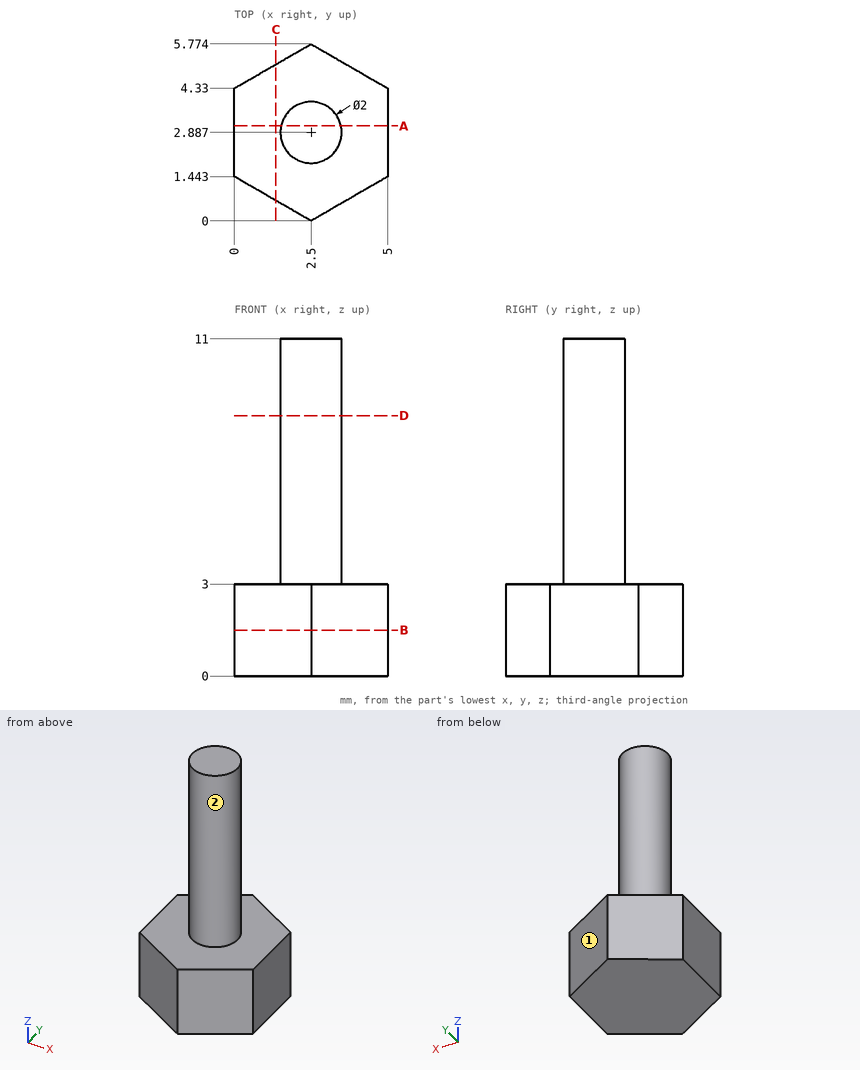
Input: dimensioned drawing with shaded views. Units: mm. Origin: part minimum x, y, z. A direction names the side the tool comes from. Give positions to 0.01 mm unless a question says otherwise; leave off trailing zeros. Order: outer loops, then holes, each group sorted by start corner. A loop starts at its lowest first (then second) coordinate and runs counter-clockwise, first axis right, second up. Notation, with made-up numbers: (-38, 70.5) -> (12, 70.5) arc R12 ccw to (12, 89.5) -> close; hole circle Ø3 at (-37.5, -15). An arc over 180 degrees is marked (long way). Answer as a JSON object with one key per item and string values.
Q1. Section D-D (z = 8.5). Output: boundary loops of the cut face in (x, y).
Entries:
{"outline": "circle Ø2 at (2.5, 2.89)"}
Q2. Section B-B (z = 1.5). Output: boundary loops of the cut face in (x, y).
Entries:
{"outline": "(0, 1.44) -> (2.5, 0) -> (5, 1.44) -> (5, 4.33) -> (2.5, 5.77) -> (0, 4.33) -> close"}
Q3. Access query for the marked faces 1 and 2. Directions: +Z, -Z, +X, -X, +Y, -Y. A direction counts if a zero-diameter tool reaches every point of the face in a straight line with its end or side. Return the directions, or none.
Entries:
{"face 1": "+Z, -Z, +X, +Y", "face 2": "+Z"}
Q4. Material intervals for probe 1 along Z at (x, y) = (0.6, 3.15); probe 2 along X at (y, z) = (2.3, 9.75); probe 3 along X at (y, z) = (4.45, 1) (1 decimal), sorted ascending.
Entries:
{"probe 1": "z = 0 to 3", "probe 2": "x = 1.69 to 3.31", "probe 3": "x = 0.2 to 4.8"}
Q5. Section C-C (x = 1.35). Output: boundary loops of the cut face in (y, z).
Entries:
{"outline": "(0.66, 0) -> (5.11, 0) -> (5.11, 3) -> (0.66, 3) -> close"}
Q6. Section A-A (y = 3.1). Output: boundary loops of the cut face in (x, z).
Entries:
{"outline": "(0, 0) -> (5, 0) -> (5, 3) -> (3.48, 3) -> (3.48, 11) -> (1.52, 11) -> (1.52, 3) -> (0, 3) -> close"}
Q7. First-contact query: pin 1 (2 mm diameter, centred on x = 1.5, z = 5, fed in from -Y). Flat tip, straight axial feed; report the tip coordinate or a pass-through.
Entries:
{"pin 1": "stops at y = 1.89"}
